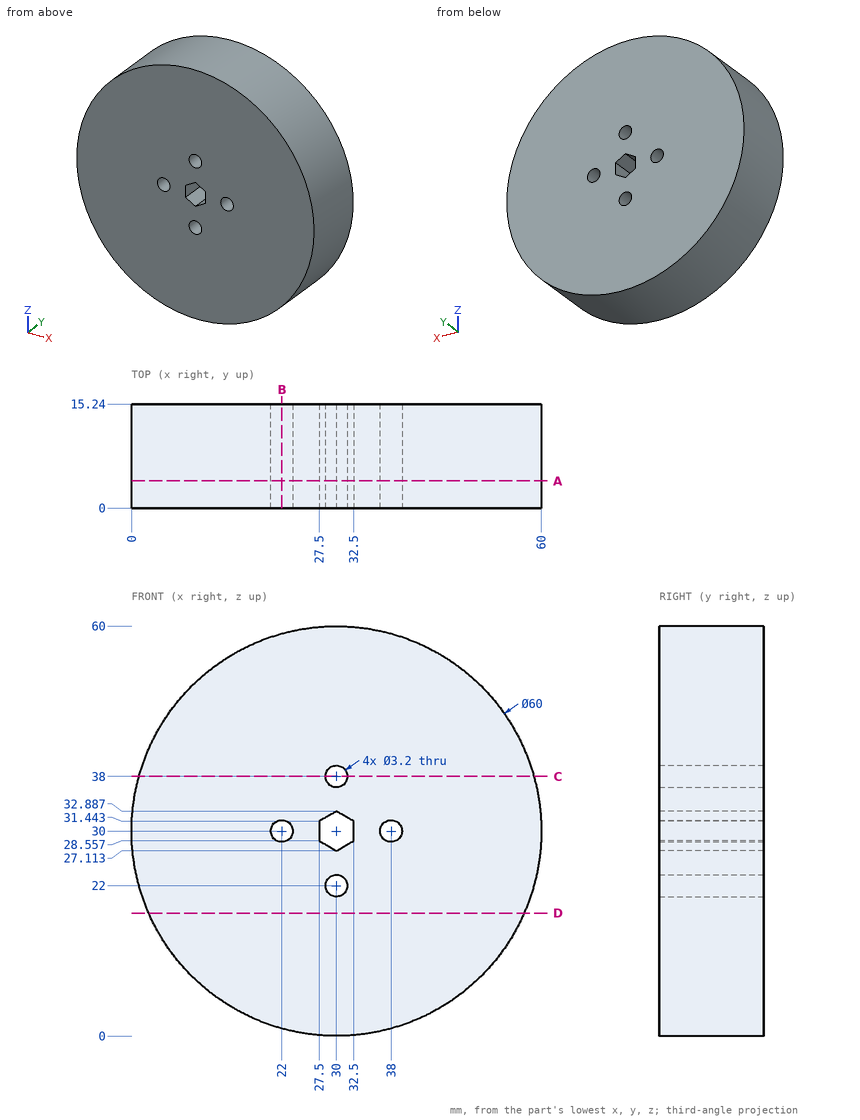
Geometry check sheet. Reference: drawing and pictorial views, mm from the part's lowest x, y, z. Give positions to 0.01 mm unless a question says otherwise; leave off trailing zeros. Loops run counter-clockwise (first coordinate to the right, second up) from the corner with the lowest first, then second, coordinate; pieces in that order, holes last. Notation, with made-up numbers: (83, -13) - (90, -13) arc R24 cw to (90, 17) - close; hole circle Ø9 at (41.5, -33.75). An arc over 180 degrees is marked (long way). Use CSV: the item, a comma, the result in double quotes. Start each with the question number.
Q1. Section check C-C, the plane z = 38. Record the cut outline in (x, y).
Q2. Section check D-D, the plane z = 18. Record the cut outline in (x, y) (1 decimal), and give its area (3 significant figures).
Q3. Section check A-A, the plane y = 4. Record the cut outline in (x, z).
Q4. Scan lines: probe 1 along Z at (x, y) = (30, 7.25); probe 2 along Z at (x, y) = (37, 2.75); probe 3 along X at (y, z) = (12.25, 38). Record each from-to range of solid material in increasing order. Write a range as from..to.
Q5. Section check B-B, the plane x = 22. Record the cut outline in (y, z).
Findings below:
1,outline,"(1.09, 0) - (28.4, 0) - (28.4, 15.24) - (1.09, 15.24) - close; (31.6, 0) - (58.91, 0) - (58.91, 15.24) - (31.6, 15.24) - close"
2,outline,"(2.5, 0) - (57.5, 0) - (57.5, 15.2) - (2.5, 15.2) - close"
2,area,"838 mm^2"
3,outline,"circle Ø60 at (30, 30); hole circle Ø3.2 at (22, 30); hole (27.5, 28.56) - (30, 27.11) - (32.5, 28.56) - (32.5, 31.44) - (30, 32.89) - (27.5, 31.44) - close; hole circle Ø3.2 at (30, 22); hole circle Ø3.2 at (30, 38); hole circle Ø3.2 at (38, 30)"
4,probe 1,"z = 0..20.4, 23.6..27.11, 32.89..36.4, 39.6..60"
4,probe 2,"z = 0.83..28.75, 31.25..59.17"
4,probe 3,"x = 1.09..28.4, 31.6..58.91"
5,outline,"(0, 1.09) - (15.24, 1.09) - (15.24, 28.4) - (0, 28.4) - close; (0, 31.6) - (15.24, 31.6) - (15.24, 58.91) - (0, 58.91) - close"
